Verification items for the finished model (mm, model axes). A direction names the side the tool comes from. Round coordinates to 2 decimals unless told otherwise and drop trailing zeros. Loops run counter-clockwise (first coordinate to the right, second up) from the corner with the lowest first, then second, coordinate; pieces in that order, holes last. Notation, with made-up numbers: M 1,48.5 L 41,48.5 A28 cw 41,77.5 Z; hole C 46.5,76.25 d5. An arc over 180 degrees is marked long. One line per item, written item: value.
from build123d import *

# Parameters (mm, degrees)
F0_W     = 45
F0_H     = 20.5
F1_DEPTH = 3
F2_R     = 8
F3_DEPTH = 12.5
F4_W     = 11
F4_H     = 3
F5_DEPTH = 4
F6_W     = 9
F6_H     = 19
F7_DEPTH = 6


with BuildPart() as f1:
    # F0 (on Front) → F1 (new body)
    with BuildSketch(Plane.XZ):
        Rectangle(F0_W, F0_H)
    extrude(amount=-F1_DEPTH)

    # F2 (on Front) → F3 (join)
    with BuildSketch(Plane.XZ):
        with Locations((-13, 0)):
            Circle(F2_R)
        with Locations((13, 0)):
            Circle(F2_R)
    extrude(amount=F3_DEPTH)

    # F4 (on Front) → F5 (join)
    with BuildSketch(Plane.XZ):
        with Locations((0, 6.75)):
            Rectangle(F4_W, F4_H)
    extrude(amount=F5_DEPTH)

    # F6 (on Front) → F7 (join)
    with BuildSketch(Plane.XZ):
        with Locations((0, -19.75)):
            Rectangle(F6_W, F6_H)
    extrude(amount=-F7_DEPTH)


solid = f1.part
(1) Tool access check on faces 4 (the face through (0, 4, -10.25)), 5 (the face through (13, 1, -10.25)), 6 (the face through (-14, 1, -10.25)), 7 (the face through (5.5, -2, 7)), 8 (the face through (11.27, -6.16, -7.81)). Record the directions out of +Z, -Z, +X, -X, +Y, -Y that give a thin tool (end or side, any length) a straight path to the whole face; none if there is none.
Completed:
face 4: +Z, +X, -X, +Y
face 5: -Z, +X, +Y, -Y
face 6: -Z, -X, +Y, -Y
face 7: +Z, -Y
face 8: -Y
(2) Mould release check, pull along X, two halves, no side actions. Record for faces 1 (the face through (0, 1, 10.25)), 2 (the face through (0, -2, 5.25)), 3 (the face through (-4.5, 3, -20)): +X half, -X half, draft (parallel to the pull), parting line (faces both ways), or undercut.
Completed:
face 1: draft
face 2: undercut
face 3: -X half
(3) Sectioned sample at B-B on z = 0. Enter the section's corners in (x, y), and give its area (3 significant figures).
Completed:
outline: M -22.5,0 L -21,0 L -21,-12.5 L -5,-12.5 L -5,0 L 5,0 L 5,-12.5 L 21,-12.5 L 21,0 L 22.5,0 L 22.5,3 L -22.5,3 Z
area: 535 mm^2
(4) Sectioned sample at D-D on x = -1. Enter the section's corners in (y, z), and give its area (4 significant figures).
Completed:
outline: M -4,5.25 L 0,5.25 L 0,-29.25 L 6,-29.25 L 6,-10.25 L 3,-10.25 L 3,10.25 L 0,10.25 L 0,8.25 L -4,8.25 Z
area: 187.5 mm^2
(5) Sectioned sample at A-A on x = 13. Enter the section's corners in (y, z), and give its area (4 significant figures).
Completed:
outline: M -12.5,-8 L 0,-8 L 0,-10.25 L 3,-10.25 L 3,10.25 L 0,10.25 L 0,8 L -12.5,8 Z
area: 261.5 mm^2
(6) Sectioned sample at C-C on y = -7.25. Enter the section's corners in (x, z), and give its area (3 significant figures).
Completed:
outline: C -13,0 d16; C 13,0 d16
area: 402 mm^2
(7) Depth check by flat-ended pin: pin 1 Ø1.5 at (x, y) = (12.5, 1.5) entering from -Z; pin 2 Ø2 at (x, z) = (2.5, -7) entering from +Y; pin 3 Ø0.9 at (x, z) = (0.5, 6.5) entering from -Y. Enter the tip coordinate at first touch or a pass-through.
Completed:
pin 1: stops at z = -10.25
pin 2: stops at y = 3
pin 3: stops at y = -4
(8) Thickness scan on L1, parallel to Y at x = -11.5, z = -9; L2, parallel to Z at x = 6.5, y = 0.75; L3, parallel to Y at x = -17.5, z = -2. Record the ranges inside material, lowest first. Write a range as from..to.
Completed:
L1: y = 0..3
L2: z = -10.25..10.25
L3: y = -12.5..3
